Autodesk Inventor part; units mm, degrees
ref_plane "YZ Plane" through (0, 0, 0) normal (1, 0, 0) x (0, 1, 0)
ref_plane "XZ Plane" through (0, 0, 0) normal (0, 1, 0) x (-1, 0, 0)
ref_plane "XY Plane" through (0, 0, 0) normal (0, 0, 1) x (1, 0, 0)
sketch "Sketch_1" plane through (0, 0, 0) normal (0, 0, 1) x (1, 0, 0)
  line L0 (-60, 40) -> (-60, 0)
  line L1 (-60, 0) -> (60, 0)
  line L2 (60, 0) -> (60, 40)
  line L3 (60, 40) -> (20, 120)
  line L4 (20, 120) -> (-20, 120)
  line L5 (-20, 120) -> (-60, 40)
  circle A0 centre (40, 20) radius 4.165
  circle A1 centre (0, 60) radius 4.165
  circle A2 centre (0, 100) radius 4.165
  circle A3 centre (0, 20) radius 4.165
  circle A4 centre (-40, 20) radius 4.165
extrude "Extrusion1" add sketch "Sketch_1" along normal blind 6
properties part number "40-4340"
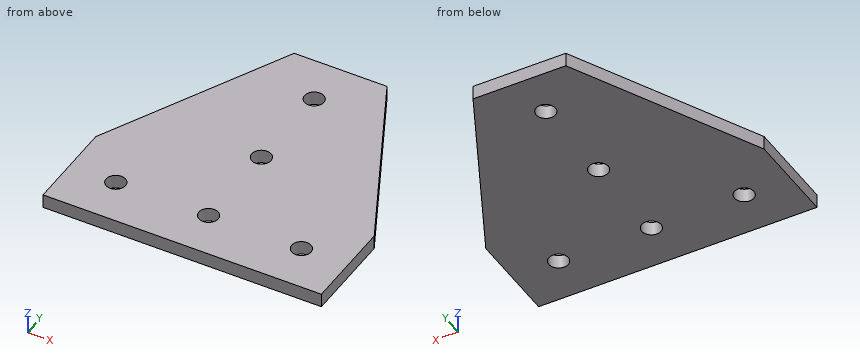
The listing builds one solid part. Answer for the finished solid, in the listing's coordinates (mm). Coordinates: 2 decimals unless noted, no trailing zeros. Order: outer loops, then holes, each group sorted by start corner. A loop starts at its lowest first (then second) coordinate and runs counter-clockwise, first axis right, second up. Notation, with made-up numbers: M 61.5,55 L 104.5,55 A19 ccw 104.5,71 Z; hole C 18,-21.75 d5. An arc over 180 degrees is marked long. Answer as a JSON object with one key per item and string values. Group by question number.
1. Section B-B on x = 0 is taken. Write down the section's boundary in (y, z) (3 decimals).
2. Section A-A on y = 20 is taken. Write down the section's boundary in (x, z) (3 decimals).
3. Section D-D on x = 40 is taken. Write down the section's boundary in (y, z) (3 decimals), then the cut area to 3 significant figures.
4. Straight lines are drawn through the part: line 1 (Y direction, x = 0, z = 3.7) (3 decimals); line 2 (X direction, y = 22.5, z = 4.2); line 3 (Y direction, x = -1, z = 4.1). For each, find the intervals that lie inside material, in ascending order.
5. Section C-C on y = 100 is taken. Write down the section's boundary in (x, z) (3 decimals), then the cut area to 3 significant figures.
6. Flat-ended cylindrical pins translate along their axes: P1, Ø6.5, axis at x = -40, y = 20, coming from the -Z side; P2, Ø1.5, axis at y = 76.5, z = 3.5, coming from the -X side (3 decimals). Find the tip coordinate at first contact, or state that the pin passes through.
Values follow:
{
 "1": {"outline": "M 0,0 L 15.835,0 L 15.835,6 L 0,6 Z; M 24.165,0 L 55.835,0 L 55.835,6 L 24.165,6 Z; M 64.165,0 L 95.835,0 L 95.835,6 L 64.165,6 Z; M 104.165,0 L 120,0 L 120,6 L 104.165,6 Z"},
 "2": {"outline": "M -60,0 L -44.165,0 L -44.165,6 L -60,6 Z; M -35.835,0 L -4.165,0 L -4.165,6 L -35.835,6 Z; M 4.165,0 L 35.835,0 L 35.835,6 L 4.165,6 Z; M 44.165,0 L 60,0 L 60,6 L 44.165,6 Z"},
 "3": {"outline": "M 0,0 L 15.835,0 L 15.835,6 L 0,6 Z; M 24.165,0 L 80,0 L 80,6 L 24.165,6 Z", "area": "430 mm2"},
 "4": {"line 1": "0 to 15.835, 24.165 to 55.835, 64.165 to 95.835, 104.165 to 120", "line 2": "-60 to -43.33, -36.67 to -3.33, 3.33 to 36.67, 43.33 to 60", "line 3": "0 to 15.96, 24.04 to 55.96, 64.04 to 95.96, 104.04 to 120"},
 "5": {"outline": "M -30,0 L -4.165,0 L -4.165,6 L -30,6 Z; M 4.165,0 L 30,0 L 30,6 L 4.165,6 Z", "area": "310 mm2"},
 "6": {"P1": "through", "P2": "x = -42.125"}
}
